Design review of the part built by this model. Coordinates are the model's own, in mm. A direction names the side the tool comes from. Coordinates: 2 decimals unless noted, no trailing zeros. Loops run counter-clockwise (first coordinate to the right, second up) from the corner with the lowest first, then second, coordinate; pieces in that order, holes last. Notation, with made-up numbers: (-37.75, 5.25) -> (-25.75, 5.25) arc R19 cw to (-25.75, 20.25) -> close; hole circle Ø6 at (81, 68). An arc over 180 degrees is marked (long way). Use CSV: the item, a comma, the result in double quotes.
```python
from build123d import *

# Parameters (mm, degrees)
F0_W     = 2
F0_H     = 15
F1_DEPTH = 5
F2_SIZE  = 0.5
F3_W     = 0.3
F3_H     = 1
F4_DEPTH = 25
F5_R     = 2


with BuildPart() as f1:
    # F0 (on Top) → F1 (new body)
    with BuildSketch(Plane.XY):
        Polygon((6.203948, 24.292763), (-6.796052, 24.292763), (-6.796052, 4.292763), (-4.796052, 4.292763), (4.203948, 4.292763), (6.203948, 4.292763), align=None)
        with Locations((-5.796052, -3.207237)):
            Rectangle(F0_W, F0_H)
        with Locations((5.203948, -3.207237)):
            Rectangle(F0_W, F0_H)
    extrude(amount=F1_DEPTH)

    # F2
    f2_edges = [f1.edges().sort_by_distance(p)[0] for p in [
        (-6.796052, -10.707237, 2.5),
        (4.203948, -10.707237, 2.5),
        (6.203948, -10.707237, 2.5),
        (-4.796052, -10.707237, 2.5),
    ]]
    chamfer(f2_edges, length=F2_SIZE)

    # F3 (on face) → F4 (cut)
    with BuildSketch(Plane.XY.offset(5)):
        with Locations((-4.946052, -7.707237)):
            Rectangle(F3_W, F3_H)
        with Locations((4.353948, -7.707237)):
            Rectangle(F3_W, F3_H)
    extrude(amount=-F4_DEPTH, mode=Mode.SUBTRACT)

    # F5
    f5_edges = [f1.edges().sort_by_distance(p)[0] for p in [
        (6.203948, 24.292763, 2.5),
        (-6.796052, 24.292763, 2.5),
    ]]
    fillet(f5_edges, radius=F5_R)


solid = f1.part
```
Item 1: To check wall thickness, follow line 1 along X through (y, z) = (-9, 1.8); line 2 along Y through (x, z) = (-3, 4.3); line 3 along Y through (x, z) = (-5, 2.55). State the ranges of each line that lie inside material, in increasing order.
Checked values:
line 1,"-6.8 to -4.8, 4.2 to 6.2"
line 2,"4.29 to 24.29"
line 3,"-10.41 to -8.21, -7.21 to 24.28"
Item 2: Add section A-A (y = -6). Give the boundary of the cut face in (x, z), then the cut area to 3 significant figures.
Checked values:
outline,"(-6.8, 0) -> (-4.8, 0) -> (-4.8, 5) -> (-6.8, 5) -> close; (4.2, 0) -> (6.2, 0) -> (6.2, 5) -> (4.2, 5) -> close"
area,"20.0 mm^2"
Item 3: Clearance check with a flat-ended pin moving along its axis: pin 1 (2.5 mm diameter, centred on x = -2.5, z = 3, fed in from -Y). State where the tip first meets the part, or that it passes through.
Checked values:
pin 1,"y = 4.29"
Item 4: Draft analysis for pull direction Y (two halves, no side actions). For faces 1 (the face through (-6.226, 23.691, 2.535)), 2 (the face through (6.204, 6, 2)), 3 (the face through (-5.096, -8, 3)), state which applies: pulls with the +Y half, pulls with the -Y half, needs draft (parallel to the pull), parting line crosses it, or undercut.
Checked values:
face 1,"pulls with the +Y half"
face 2,"needs draft"
face 3,"undercut"
Item 5: Machinability: for faces 4 (the face through (4.204, -9, 2)), 5 (the face through (-6, -10.707, 2)), 6 (the face through (4.504, -8, 3)), which of the approach directions +Z, -Z, +X, -X, +Y, -Y give a long, thin tool a straight path to every point of the face, cutting with its end or side? Answer none if there is none.
Checked values:
face 4,"+Z, -Z, -Y"
face 5,"+Z, -Z, +X, -X, -Y"
face 6,"+Z, -Z"
Item 6: Add section C-C (x = 0.25). Give the boundary of the cut face in (y, z), then the cut area to 3 significant figures.
Checked values:
outline,"(4.29, 0) -> (24.29, 0) -> (24.29, 5) -> (4.29, 5) -> close"
area,"100 mm^2"
Item 7: Add section B-B (z = 4.35). Give the boundary of the cut face in (x, y), then the cut area to 3 significant figures.
Checked values:
outline,"(-6.8, -10.21) -> (-6.3, -10.71) -> (-5.3, -10.71) -> (-4.8, -10.21) -> (-4.8, -8.21) -> (-5.1, -8.21) -> (-5.1, -7.21) -> (-4.8, -7.21) -> (-4.8, 4.29) -> (4.2, 4.29) -> (4.2, -7.21) -> (4.5, -7.21) -> (4.5, -8.21) -> (4.2, -8.21) -> (4.2, -10.21) -> (4.7, -10.71) -> (5.7, -10.71) -> (6.2, -10.21) -> (6.2, 22.29) arc R2 ccw to (4.2, 24.29) -> (-4.8, 24.29) arc R2 ccw to (-6.8, 22.29) -> close"
area,"317 mm^2"
